Autodesk Inventor part; units mm, degrees
ref_plane "YZ Plane" through (0, 0, 0) normal (1, 0, 0) x (0, 1, 0)
ref_plane "XZ Plane" through (0, 0, 0) normal (0, 1, 0) x (-1, 0, 0)
ref_plane "XY Plane" through (0, 0, 0) normal (0, 0, 1) x (1, 0, 0)
sketch "Sketch1" plane through (0, 0, 0) normal (0, 1, 0) x (-1, 0, 0)
  circle A0 centre (0, 0) radius 106
  dimension "d1" = 212
extrude "Extrusion1" add sketch "Sketch1" along normal mid plane 6.35
sketch "Sketch2" plane through (0, 3.175, 0) normal (0, 1, 0) x (1, 0, 0)
  circle A0 centre (0, 22.5) radius 2.05
  circle A1 centre (-15.9099, 15.9099) radius 2.05
  circle A2 centre (-22.5, 0) radius 2.05
  circle A3 centre (-15.9099, -15.9099) radius 2.05
  circle A4 centre (0, -22.5) radius 2.05
  circle A5 centre (15.9099, -15.9099) radius 2.05
  circle A6 centre (22.5, 0) radius 2.05
  circle A7 centre (15.9099, 15.9099) radius 2.05
  point P0 (0, 0)
  dimension "d4" = 4.1
  dimension "d5" = 22.5
  dimension "d8" = 360
extrude "Extrusion2" cut sketch "Sketch2" against normal through all
sketch "Sketch3" plane through (0, 3.175, 0) normal (0, 1, 0) x (1, 0, 0)
  circle A0 centre (0, 0) radius 16.1
  dimension "d12" = 32.2
extrude "Extrusion3" cut sketch "Sketch3" against normal through all
sketch "Sketch8" plane through (0, 3.175, 0) normal (0, 1, 0) x (1, 0, 0)
  circle A0 centre (-26, -54) radius 2.1
  circle A1 centre (0, 0) radius 106 construction
  line L0 (0, -106) -> (0, 0) construction
  circle A2 centre (-26, -42) radius 2.1
  circle A3 centre (-26, -30) radius 2.1
  circle A4 centre (-26, -18) radius 2.1
  circle A5 centre (-26, -6) radius 2.1
  circle A6 centre (-26, 6) radius 2.1
  circle A7 centre (-26, 18) radius 2.1
  circle A8 centre (-26, 30) radius 2.1
  circle A9 centre (-26, 42) radius 2.1
  circle A10 centre (-26, 54) radius 2.1
  line L1 (-26, -6) -> (-26, 6) construction
  circle A11 centre (-72, -54) radius 2.1
  circle A12 centre (-72, -42) radius 2.1
  circle A13 centre (-72, -30) radius 2.1
  circle A14 centre (-72, -18) radius 2.1
  circle A15 centre (-72, -6) radius 2.1
  circle A16 centre (-72, 6) radius 2.1
  circle A17 centre (-72, 18) radius 2.1
  circle A18 centre (-72, 30) radius 2.1
  circle A19 centre (-72, 42) radius 2.1
  circle A20 centre (-72, 54) radius 2.1
  point P0 (-26, 0)
  dimension "d71" = 4.2
  dimension "d74" = 12
  dimension "d79" = 26
  dimension "d80" = 4.2
  dimension "d83" = 12
  dimension "d88" = 46
extrude "Extrusion7" cut sketch "Sketch8" against normal through all contours A0 | A2 | A3 | A4 | A7 | A8 | A9 | A10 | A11 | A12 | A13 | A14 | A15 | A16 | A17 | A18 | A19 | A20
sketch "Sketch9" plane through (0, 3.175, 0) normal (0, 1, 0) x (1, 0, 0)
  circle A0 centre (60, -42) radius 2.1
  line L0 (0, 0) -> (0, 16.1) construction
  circle A1 centre (0, 0) radius 16.1 construction
  line L1 (0, 0) -> (16.1, 0) construction
  circle A2 centre (60, -28) radius 2.1
  circle A3 centre (60, -14) radius 2.1
  circle A4 centre (60, 0) radius 2.1
  circle A5 centre (60, 14) radius 2.1
  circle A6 centre (60, 28) radius 2.1
  circle A7 centre (60, 42) radius 2.1
  circle A8 centre (92, -42) radius 2.1
  circle A9 centre (92, -28) radius 2.1
  circle A10 centre (92, -14) radius 2.1
  circle A11 centre (92, 0) radius 2.1
  circle A12 centre (92, 14) radius 2.1
  circle A13 centre (92, 28) radius 2.1
  circle A14 centre (92, 42) radius 2.1
  dimension "d91" = 4.2
  dimension "d92" = 60
  dimension "d93" = 42
  dimension "d96" = 14
  dimension "d99" = 32
extrude "Extrusion8" cut sketch "Sketch9" against normal through all
properties part number "ArmBase" material "Aluminum 6061"
Source: CAD feature listing. Evaluate the final solid. Frame: model axes, mm. Round coordinates to 2 decimals unless told otherwise and drop trailing zeros. Loops run counter-clockwise (first coordinate to the right, second up) from the corner with the lowest first, then second, coordinate; pieces in that order, holes last. Notation, with made-up numbers: M 21,79.5 L 41,79.5 A18 cw 41,86.5 Z; hole C 14,52.25 d5. An arc over 180 degrees is marked long. Put each result on its own line as item: value.
(1) Section A-A, the plane y = 1.25. State how many separate pieces and enclosed holes the cut face has, and give its area (3 significant figures).
Solutions:
separate pieces: 1
enclosed holes: 41
area: 33,900 mm²
(2) Section C-C, the plane z = 73. Return loops of the section in (x, y) (3 decimals), and give its area (3 significant figures).
Solutions:
outline: M -76.857,-3.175 L 76.857,-3.175 L 76.857,3.175 L -76.857,3.175 Z
area: 976 mm²
(3) Section B-B, the plane x = 28. Return loops of the section in (y, z) (3 decimals).
Solutions:
outline: M -3.175,-102.235 L 3.175,-102.235 L 3.175,102.235 L -3.175,102.235 Z
(4) First-contact query: pin 1 (4.5 mm diameter, centred on x = 0, z = 22.5, fed in from -Y) (3 decimals); pin 2 (3.5 mm diameter, centred on x = 60, z = 28, fed in from +Y); pin 3 (1.5 mm diameter, centred on x = -83.5, y = 1.5, fed in from +Z); pin 4 (2 mm diameter, centred on x = 62.5, y = -1.5, fed in from +Z). Flat tips, straight axial feed; report the tip coordinate or a pass-through.
Solutions:
pin 1: y = -3.175
pin 2: through
pin 3: z = 66.25
pin 4: z = 86.34
(5) Pull-direction query (Z, two-part tool) for faces 1 (the face through (-56.985, -0.044, -89.38)), 2 (the face through (1, -3.175, 25)), 3 (the face through (15.357, 0.044, -4.836)); classes: released by +Z, released by -Z, zero draft, split by the parting line, or undercut.
Solutions:
face 1: split by the parting line
face 2: zero draft
face 3: undercut
(6) Ray query, line 1 (Z direction, x = 0, y = -1.5); line 2 (X direction, y = 1.5, z = -54); line 3 (Z direction, x = -14.5, y = 2.25). Return the intervals inside material, ascending. Write a range as [from, to].
Solutions:
line 1: [-106, -24.55], [-20.45, -16.1], [16.1, 20.45], [24.55, 106]
line 2: [-91.21, -74.1], [-69.9, -28.1], [-23.9, 91.21]
line 3: [-105, -17.4], [-14.42, -7], [7, 14.42], [17.4, 105]
